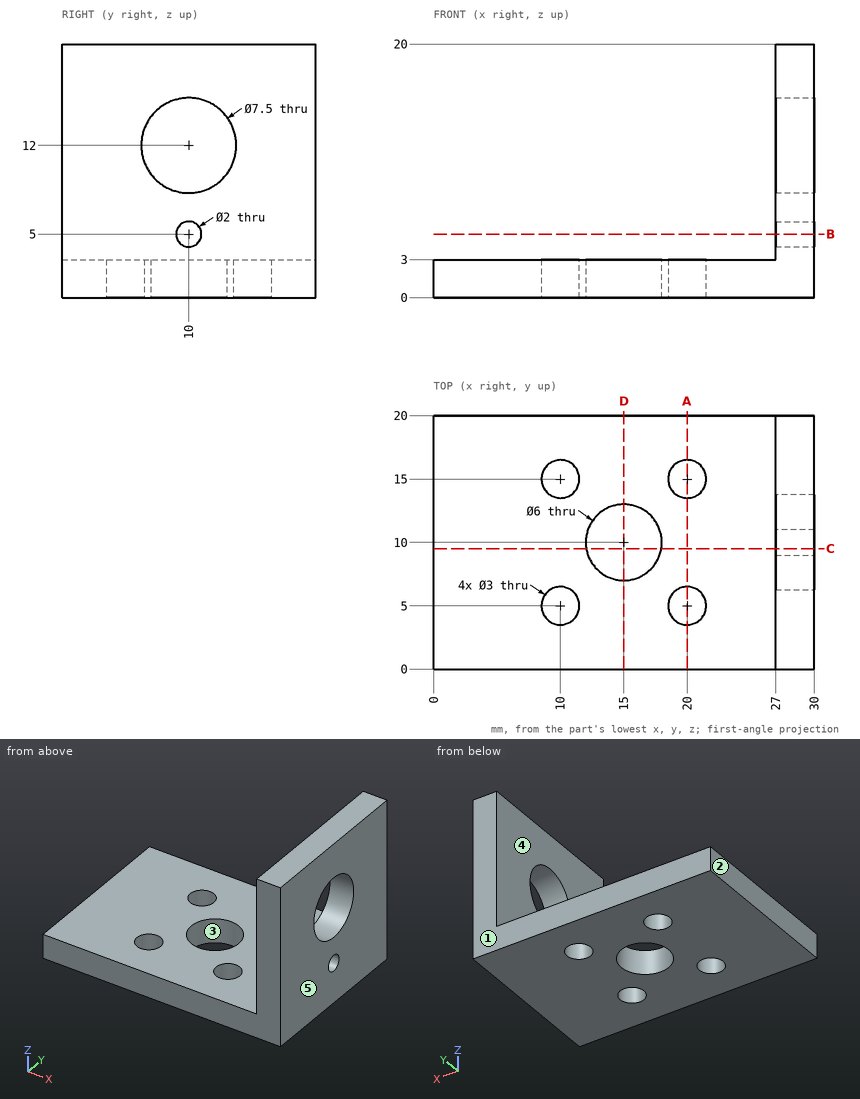
Here's the drawing with two shaded views (mm, measured from the low corner). I have some questions. A direction names the side the tool comes from. Give positions to 0.01 mm unless a question says otherwise; leave off trailing zeros. Write each loop counter-clockwise with the first axis right and the second up, starting at its lowest first coordinate (ties: lowest second). Pieces come first, ordered by that corner, then holes. Notation, with made-up numbers: (81.25, 29) -> (92.25, 29) arc R17 ccw to (92.25, 53) -> close; hole circle Ø8 at (19, 36.25). An arc over 180 degrees is marked (long way). Use one line per item in the form item = value.
1) On a 3-axis mill with a long thin cutter (end or side, diameter ignored), from which of +Z, -Z, +X, -X, +Y, -Y can I reach the whole of each face in a straight line? I mean the marked faces 4 and 5. Say none if no direction works.
Verdict:
face_4 = +Z, -X, +Y, -Y
face_5 = +Z, -Z, +X, +Y, -Y
2) I'm going to push flat-ended pins straight in: pin 1 (2.5 mm diameter, centred on x = 20, y = 5, fed in from -Z); pin 2 (1.5 mm diameter, centred on y = 18, z = 10, fed in from -X); pin 3 (3.5 mm diameter, centred on x = 10, y = 5, fed in from +Z). Where does each tip first touch, or does it pass through?
Verdict:
pin_1 = through
pin_2 = 27
pin_3 = 3
3) Suppose I cut it at B-B (z = 5). Please give me the cut outline in (x, y), and give its area (3 significant figures).
Verdict:
outline = (27, 0) -> (30, 0) -> (30, 9) -> (27, 9) -> close; (27, 11) -> (30, 11) -> (30, 20) -> (27, 20) -> close
area = 54.0 mm2
4) Suppose I cut it at A-A (x = 20). Please give me the cut outline in (y, z), and give its area (3 significant figures).
Verdict:
outline = (0, 0) -> (3.5, 0) -> (3.5, 3) -> (0, 3) -> close; (6.5, 0) -> (13.5, 0) -> (13.5, 3) -> (6.5, 3) -> close; (16.5, 0) -> (20, 0) -> (20, 3) -> (16.5, 3) -> close
area = 42.0 mm2
5) If I drill on L1, parallel to Y at x = 10, z = 2.4; L2, parallel to Z at x = 27.6, y = 10; L3, parallel to X at y = 16, z = 1, over which ranges is the centre line in solid material (lowest first)? Write a range as [from, to].
Verdict:
L1 = [0, 3.5], [6.5, 13.5], [16.5, 20]
L2 = [0, 4], [6, 8.25], [15.75, 20]
L3 = [0, 8.88], [11.12, 18.88], [21.12, 30]
6) Suppose I cut it at D-D (x = 15). Please give me the cut outline in (y, z), and give its area (3 significant figures).
Verdict:
outline = (0, 0) -> (7, 0) -> (7, 3) -> (0, 3) -> close; (13, 0) -> (20, 0) -> (20, 3) -> (13, 3) -> close
area = 42.0 mm2
7) Suppose I cut it at C-C (y = 9.5). Please give me the cut outline in (x, z), and give its area (3 significant figures).
Verdict:
outline = (0, 0) -> (12.04, 0) -> (12.04, 3) -> (0, 3) -> close; (17.96, 0) -> (30, 0) -> (30, 4.13) -> (27, 4.13) -> (27, 3) -> (17.96, 3) -> close; (27, 5.87) -> (30, 5.87) -> (30, 8.28) -> (27, 8.28) -> close; (27, 15.72) -> (30, 15.72) -> (30, 20) -> (27, 20) -> close
area = 95.8 mm2
8) We'd pull the mould along Y, two halves only. Please class the marked faces 1, 2 and 3: +Y half, -Y half, draft (parallel to the pull), parting line (faces both ways), or undercut.
Verdict:
face_1 = +Y half
face_2 = draft
face_3 = undercut
